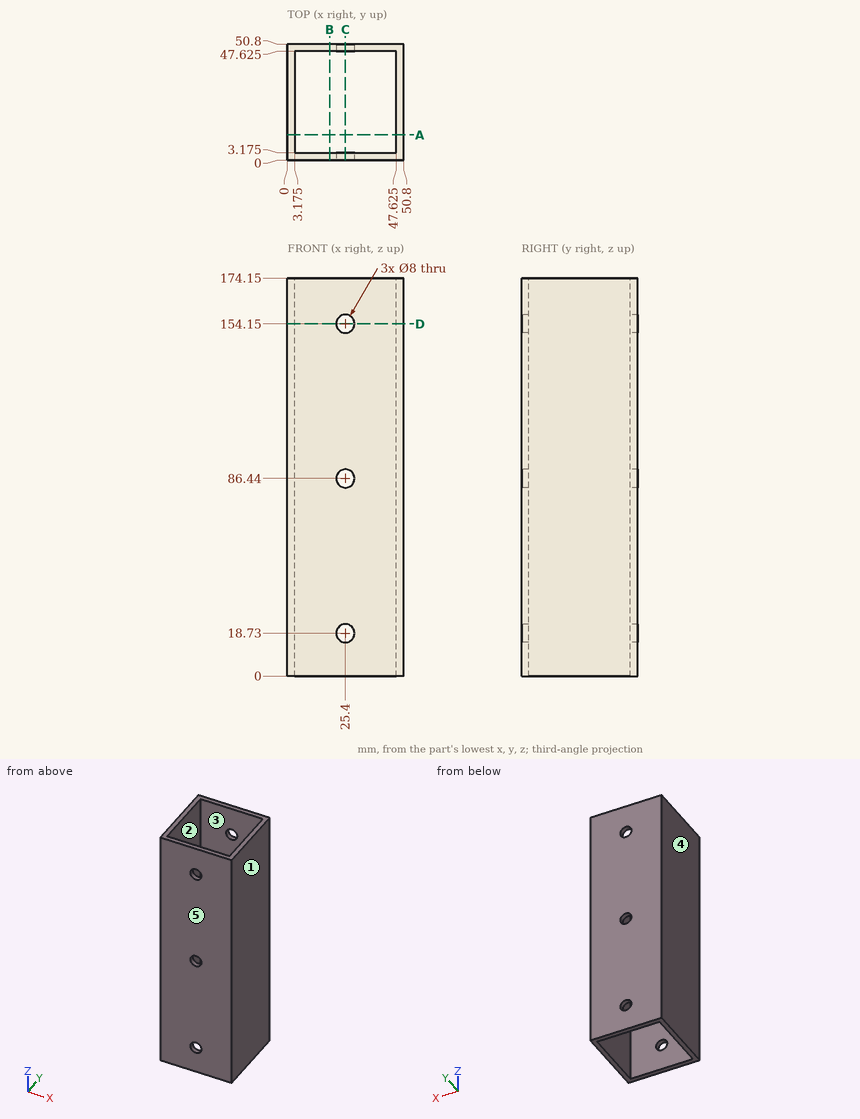
For this review, use the dimensioned drawing (mm, ordinates from the lowest corner) and the shaded views. A direction names the side the tool comes from. Coordinates: 2 decimals unless noted, no trailing zeros. Loops run counter-clockwise (first coordinate to the right, second up) from the corner with the lowest first, then second, coordinate; pieces in that order, holes last.
1. Add section A-A, the plane y = 11. Give the boundary of the cut face in (x, z) (3 decimals).
2. Add section C-C, the plane x = 25.4. Count the separate pieces of the cut face and the enclosed holes in it, then the cut area to 3 significant figures.
3. Add section D-D, the plane z = 154.15. Give the boundary of the cut face in (x, y) (3 decimals), then the cut area to 3 significant figures.
4. Mouldability with a two-part tool opening along X and no side actions: class the marked faces 3, 4 and 5 as +X half, -X half, draft (parallel to the pull), parting line (faces both ways), or undercut.
5. For the marked faces 1 and 2, list the 3-axis set-ups (+Z, -Z, +X, -X, +Y, -Y) from which the entire face can be reached by the end or side of a thin tool; tool diameter is ignored.
6. For line 1 (Z direction, x = 25.4, y = 2.4); line 2 (X direction, y = 34.5, z = 167.5) (3 decimals), list the stretches that pass through material, from the lowest coordinate up.
Result:
1. outline: (0, 0) - (3.175, 0) - (3.175, 174.15) - (0, 174.15) - close; (47.625, 0) - (50.8, 0) - (50.8, 174.15) - (47.625, 174.15) - close
2. separate pieces: 8
2. enclosed holes: 0
2. area: 953 mm2
3. outline: (0, 0) - (21.4, 0) - (21.4, 3.175) - (3.175, 3.175) - (3.175, 47.625) - (21.4, 47.625) - (21.4, 50.8) - (0, 50.8) - close; (29.4, 0) - (50.8, 0) - (50.8, 50.8) - (29.4, 50.8) - (29.4, 47.625) - (47.625, 47.625) - (47.625, 3.175) - (29.4, 3.175) - close
3. area: 554 mm2
4. face 3: undercut
4. face 4: -X half
4. face 5: draft
5. face 1: +Z, -Z, +X, +Y, -Y
5. face 2: +Z, -Z
6. line 1: z = 0 to 14.73, 22.73 to 82.44, 90.44 to 150.15, 158.15 to 174.15
6. line 2: x = 0 to 3.175, 47.625 to 50.8
